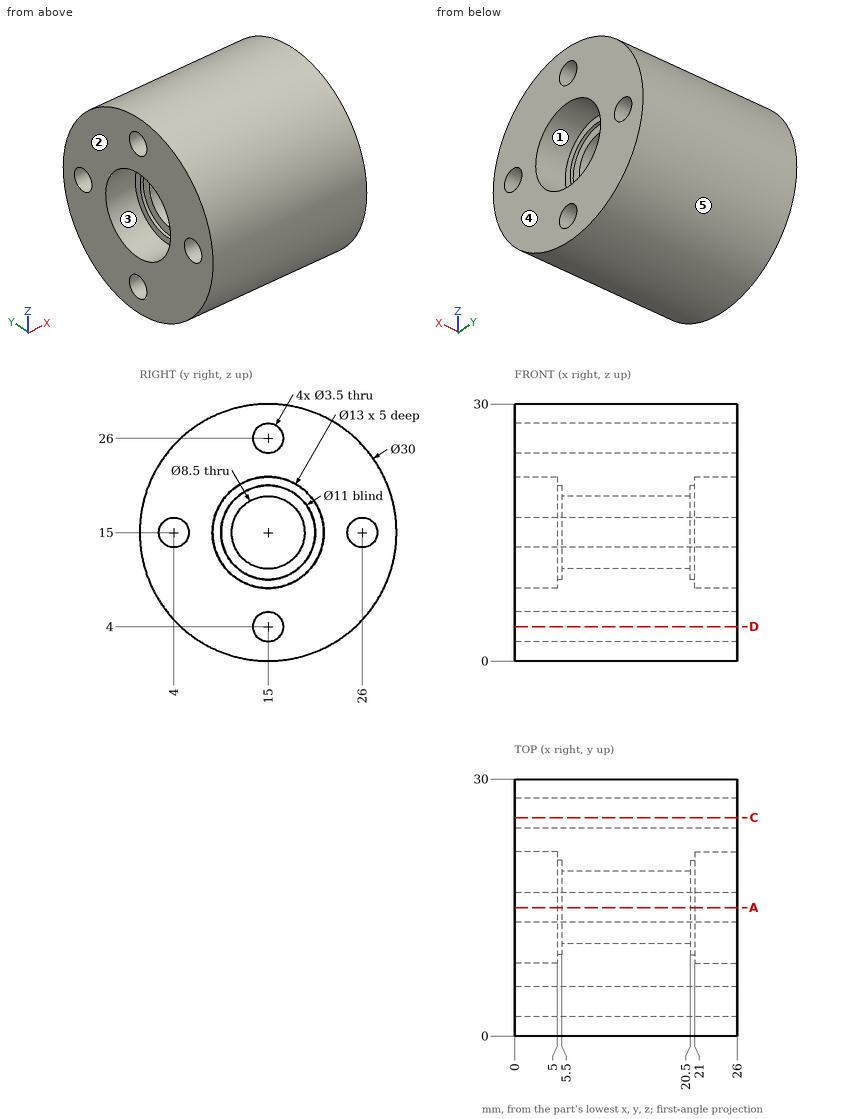
Input: dimensioned drawing with shaded views. Units: mm. Origin: part minimum x, y, z. A direction names the side the tool comes from. Coordinates: 2 decimals unless noted, no trailing zeros. Order: outer loops, then holes, each group sorted by start corner. A loop starts at its lowest first (then second) coordinate and runs counter-clockwise, first axis right, second up. Notation, with made-up numbers: (59, 79) - (89, 79) arc R22 cw to (89, 95) - close; hole circle Ø10 at (29, 78). An arc over 180 degrees is marked (long way). One line per item, written item: value.
1) Reachability of the marked faces 1 and 2 from +Z, -Z, +X, -X, +Y, -Y: full face, straight path, thin tool, end or side. Return the list, or none.
Computed values:
face 1: +X
face 2: +Z, -Z, -X, +Y, -Y
2) Cut plane D-D on z = 4. Output: boundary loops of the cut face in (x, y).
Computed values:
outline: (0, 4.8) - (26, 4.8) - (26, 13.25) - (0, 13.25) - close; (0, 16.75) - (26, 16.75) - (26, 25.2) - (0, 25.2) - close
3) Cut plane A-A on y = 15. State how many separate pieces and enclosed holes the cut face has, plus the area to 4 significant figures.
Computed values:
separate pieces: 4
enclosed holes: 0
area: 329.5 mm^2
4) Contact query for flat-ended pins moving along their axis: pin 1 (9 mm diameter, centred on y = 15, z = 15, fed in from -X); pin 2 (8 mm diameter, centred on x = 4, y = 23, fed in from -Z); pin 3 (3 mm diameter, centred on y = 15, z = 26, fed in from -X); pin 4 (1 mm diameter, centred on x = 6, z = 4.5, fed in from +Y). Output: stop coordinate, or through.
Computed values:
pin 1: stops at x = 5.5
pin 2: stops at z = 0.54
pin 3: passes through
pin 4: stops at y = 26.18
5) Mould query, pull axis Y, two halves, no side actions, for the marked faces 3, 4 and 5. Classes: released by +Y, released by -Y, zero draft, split by the parting line, or undercut.
Computed values:
face 3: undercut
face 4: zero draft
face 5: split by the parting line
6) Ray query, line 1 (Z direction, x = 8.5, y = 15); line 2 (Z direction, x = 15.5, y = 16.5); line 3 (Z direction, x = 3.5, y = 11.5). Return the intervals inside material, ascending. Write a range as [from, to].
Computed values:
line 1: z = [0, 2.25], [5.75, 10.75], [19.25, 24.25], [27.75, 30]
line 2: z = [0.08, 3.1], [4.9, 11.02], [18.98, 25.1], [26.9, 29.92]
line 3: z = [0.41, 9.52], [20.48, 29.59]
7) Cut plane C-C on y = 25.5. Output: boundary loops of the cut face in (x, z), plus the area to 3 significant figures.
Computed values:
outline: (0, 4.29) - (26, 4.29) - (26, 13.32) - (0, 13.32) - close; (0, 16.68) - (26, 16.68) - (26, 25.71) - (0, 25.71) - close
area: 470 mm^2
